For this review, take the finished solid that the model builds, in its own axes (mm). Round coordinates to 2 decimals unless told otherwise and drop trailing zeros. Loops run counter-clockwise (first coordinate to the right, second up) from the corner with the lowest first, then second, coordinate; pieces in that order, holes last. Notation, with made-up numbers: (-3.75, 75) -> (8.25, 75) arc R11 cw to (8.25, 82) -> close; hole circle Ø2 at (19, 81.5). An arc over 180 degrees is marked (long way). Write each question's results on one line, items separated by ' | '.
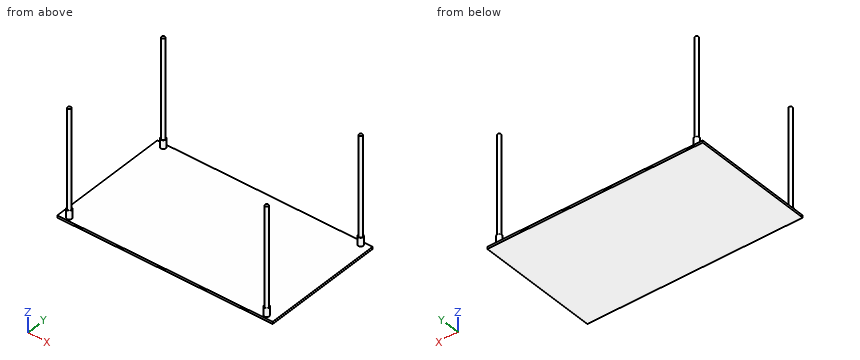
```python
from build123d import *

# Parameters (mm, degrees)
F0_W     = 100.1612991095
F0_H     = 57.3387145996
F1_DEPTH = 1
F4_R     = 0.75
F5_DEPTH = 50
F6_R     = 1.159755705
F6_R_2   = 0.9527404517
F7_DEPTH = 5


# Not quite as in the source:
# - a feature names something its author has since deleted; it is built from what else it names


with BuildPart() as f1:
    # F0 (on Top) → F1 (new body)
    with BuildSketch(Plane.XY):
        Rectangle(F0_W, F0_H)
    extrude(amount=F1_DEPTH)

    # F4 (on face) → F5 (join)
    with BuildSketch(Plane.XY.offset(1)):
        with Locations((-45.9097400308, 26.9193572998)):
            Circle(F4_R)
    extrude(amount=F5_DEPTH)

    # F6 (on Top) → F7 (join)
    with BuildSketch(Plane.XY):
        with Locations((-45.9088794887, 26.9124545157)):
            Circle(F6_R)
        with Locations((-45.9088794887, 26.9124545157)):
            Circle(F6_R_2, mode=Mode.SUBTRACT)
    extrude(amount=F7_DEPTH)

    # F8: F1 across plane


with BuildPart() as f1_1:
    add(f1.part)
    add(f1.part.mirror(Plane.XZ))

    # F9: F1 across plane


with BuildPart() as f1_2:
    add(f1_1.part)
    add(f1_1.part.mirror(Plane.YZ))


solid = f1_2.part
```
1. Consider section C-C (y = 21). State the section outline as (x, z) points.
Values found:
outline: (-50.08, 0) -> (50.08, 0) -> (50.08, 1) -> (-50.08, 1) -> close
2. Consider section A-A (z = 22). State the section outline as (x, y) points.
Values found:
outline: circle Ø1.5 at (-45.91, -26.92); circle Ø1.5 at (-45.91, 26.92); circle Ø1.5 at (45.91, -26.92); circle Ø1.5 at (45.91, 26.92)
3. For pin 1 (6 mm diameter, centred on x = -29.5, y = -3, fed in from +Z); pin 2 (12 mm diameter, centred on y = 21.5, z = 39, fed in from +X), all flat-tipped, find the tip position at first contact; note any pin that passes through.
Values found:
pin 1: stops at z = 1 | pin 2: stops at x = 46.66
4. Consider section B-B (x = -6.5). State the section outline as (y, z) points, plus the area to 3 significant figures.
Values found:
outline: (-28.67, 0) -> (28.67, 0) -> (28.67, 1) -> (-28.67, 1) -> close | area: 57.3 mm2
5. To check wall thickness, follow probe 1 along Z at (x, y) = (-28, 22.5). State the ranges of the line that lie inside material, in increasing order.
Values found:
probe 1: z = 0 to 1
